Here's how the part is built. I have some questions about the finished solid (model axes, mm). Round coordinates to 2 decimals unless told otherwise and drop trailing zeros. Loops run counter-clockwise (first coordinate to the right, second up) from the corner with the lowest first, then second, coordinate; pieces in that order, holes last. Notation, with made-up numbers: (-22.75, 50) -> (-13.75, 50) arc R17 ccw to (-13.75, 54) -> close; hole circle Ø1 at (12, 3). An arc over 180 degrees is marked (long way). Use CSV: the item, a comma, the result in double quotes. Start each with the question number.
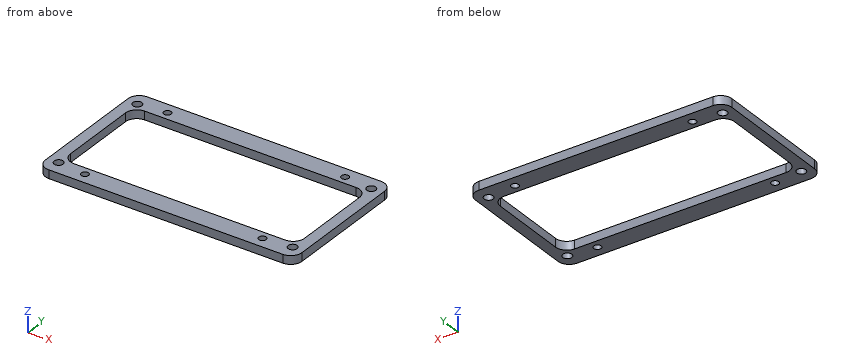
from build123d import *

# Parameters (mm, degrees)
SKETCH_1_W          = 91
SKETCH_1_H          = 50
SKETCH_1_W_2        = 83
SKETCH_1_H_2        = 36
EXTRUDE_1_DEPTH     = 3
SKETCH_2_R          = 1.3
CUT_EXTRUDE_1_DEPTH = 3
SKETCH_3_R          = 1.6
CUT_EXTRUDE_2_DEPTH = 3
FILLET_1_R          = 4
SKETCH_4_W          = 30
SKETCH_4_H          = 35
EXTRUDE_2_DEPTH     = 3
SKETCH_5_R          = 1.25
CUT_EXTRUDE_3_DEPTH = 10
FILLET_2_R          = 3
SKETCH_6_W          = 18
SKETCH_6_H          = 27
CUT_EXTRUDE_4_DEPTH = 10
FILLET_3_R          = 2
SKETCH_7_W          = 38
SKETCH_7_H          = 10
SKETCH_7_R          = 1.6
EXTRUDE_3_DEPTH     = 3
FILLET_4_R          = 2
FILLET_5_R          = 2
SKETCH_8_W          = 42
SKETCH_8_H          = 10
CUT_EXTRUDE_5_DEPTH = 10
SKETCH_9_W          = 30
SKETCH_9_H          = 41
CUT_EXTRUDE_6_DEPTH = 10


with BuildPart() as part:
    # 草图1 → 凸台-拉伸1 (new body)
    with BuildSketch(Plane.XY):
        Rectangle(SKETCH_1_W, SKETCH_1_H)
        Rectangle(SKETCH_1_W_2, SKETCH_1_H_2, mode=Mode.SUBTRACT)
    extrude(amount=EXTRUDE_1_DEPTH)

    # 草图2 → 切除-拉伸1 (cut)
    with BuildSketch(Plane.XY.offset(3)):
        with Locations((31.5, 21)):
            Circle(SKETCH_2_R)
        with Locations((31.5, -21)):
            Circle(SKETCH_2_R)
        with Locations((-31.5, -21)):
            Circle(SKETCH_2_R)
        with Locations((-31.5, 21)):
            Circle(SKETCH_2_R)
    extrude(amount=-CUT_EXTRUDE_1_DEPTH, mode=Mode.SUBTRACT)

    # 草图3 → 切除-拉伸2 (cut)
    with BuildSketch(Plane.XY.offset(3)):
        with Locations((41.5, 20)):
            Circle(SKETCH_3_R)
        with Locations((41.5, -20)):
            Circle(SKETCH_3_R)
        with Locations((-41.5, -20)):
            Circle(SKETCH_3_R)
        with Locations((-41.5, 20)):
            Circle(SKETCH_3_R)
    extrude(amount=-CUT_EXTRUDE_2_DEPTH, mode=Mode.SUBTRACT)

    # 圆角1
    fillet_1_edges = [part.edges().sort_by_distance(p)[0] for p in [
        (41.5, -18, 1.5),
        (41.5, 18, 1.5),
        (-41.5, 18, 1.5),
        (-41.5, -18, 1.5),
        (45.5, -25, 1.5),
        (-45.5, -25, 1.5),
        (-45.5, 25, 1.5),
        (45.5, 25, 1.5),
    ]]
    fillet(fillet_1_edges, radius=FILLET_1_R)

    # 草图4 → 凸台-拉伸2 (add)
    with BuildSketch(Plane(origin=(0, 0, 0), x_dir=(-1, 0, 0), z_dir=(0, 0, -1))):
        with Locations((-60.5, 0)):
            Rectangle(SKETCH_4_W, SKETCH_4_H)
    extrude(amount=-EXTRUDE_2_DEPTH)

    # 草图5 → 切除-拉伸3 (cut)
    with BuildSketch(Plane(origin=(0, 0, 0), x_dir=(-1, 0, 0), z_dir=(0, 0, -1))):
        with Locations((-70.5, -12)):
            Circle(SKETCH_5_R)
        with Locations((-70.5, 12)):
            Circle(SKETCH_5_R)
    extrude(amount=-CUT_EXTRUDE_3_DEPTH, mode=Mode.SUBTRACT)

    # 圆角2
    fillet_2_edges = [part.edges().sort_by_distance(p)[0] for p in [
        (45.5, 17.5, 1.5),
        (45.5, -17.5, 1.5),
        (75.5, -17.5, 1.5),
        (75.5, 17.5, 1.5),
    ]]
    fillet(fillet_2_edges, radius=FILLET_2_R)

    # 草图6 → 切除-拉伸4 (cut)
    with BuildSketch(Plane(origin=(0, 0, 0), x_dir=(-1, 0, 0), z_dir=(0, 0, -1))):
        with Locations((-57.5, 0)):
            Rectangle(SKETCH_6_W, SKETCH_6_H)
    extrude(amount=-CUT_EXTRUDE_4_DEPTH, mode=Mode.SUBTRACT)

    # 圆角3
    fillet_3_edges = [part.edges().sort_by_distance(p)[0] for p in [
        (66.5, -13.5, 1.5),
        (66.5, 13.5, 1.5),
        (48.5, 13.5, 1.5),
        (48.5, -13.5, 1.5),
    ]]
    fillet(fillet_3_edges, radius=FILLET_3_R)

    # 草图7 → 凸台-拉伸3 (add)
    with BuildSketch(Plane(origin=(0, 0, 0), x_dir=(-1, 0, 0), z_dir=(0, 0, -1))):
        with Locations((0, 30)):
            Rectangle(SKETCH_7_W, SKETCH_7_H)
        with Locations((-16, 32)):
            Circle(SKETCH_7_R, mode=Mode.SUBTRACT)
        with Locations((16, 32)):
            Circle(SKETCH_7_R, mode=Mode.SUBTRACT)
        with Locations((0, -30)):
            Rectangle(SKETCH_7_W, SKETCH_7_H)
        with Locations((16, -32)):
            Circle(SKETCH_7_R, mode=Mode.SUBTRACT)
        with Locations((-16, -32)):
            Circle(SKETCH_7_R, mode=Mode.SUBTRACT)
    extrude(amount=-EXTRUDE_3_DEPTH)

    # 圆角4
    fillet_4_edges = [part.edges().sort_by_distance(p)[0] for p in [
        (19, 35, 1.5),
        (-19, 35, 1.5),
        (-19, -35, 1.5),
        (19, -35, 1.5),
    ]]
    fillet(fillet_4_edges, radius=FILLET_4_R)

    # 圆角5
    fillet_5_edges = [part.edges().sort_by_distance(p)[0] for p in [
        (19, 25, 1.5),
        (-19, 25, 1.5),
        (-19, -25, 1.5),
        (19, -25, 1.5),
    ]]
    fillet(fillet_5_edges, radius=FILLET_5_R)

    # 草图8 → 切除-拉伸5 (cut)
    with BuildSketch(Plane.XY.offset(3)):
        with Locations((0, 30)):
            Rectangle(SKETCH_8_W, SKETCH_8_H)
        with Locations((0, -30)):
            Rectangle(SKETCH_8_W, SKETCH_8_H)
    extrude(amount=-CUT_EXTRUDE_5_DEPTH, mode=Mode.SUBTRACT)

    # 草图9 → 切除-拉伸6 (cut)
    with BuildSketch(Plane.XY.offset(3)):
        with Locations((60.5, 0)):
            Rectangle(SKETCH_9_W, SKETCH_9_H)
    extrude(amount=-CUT_EXTRUDE_6_DEPTH, mode=Mode.SUBTRACT)


solid = part.part
Q1. I want a section at D-D, the plane x = -29. List the corners of the cut face in (y, z) for me, then the cut area to 3 significant figures.
Q2. I want a section at C-C, the plane z = 2. Count the separate pieces of the cut face and the enclosed holes in it, then the cut area to 3 significant figures.
Q3. I want a section at B-B, the plane y = 2. List the corners of the cut face in (x, z) for me.
Q4. I want a section at A-A, the plane x = 31.5. List the corners of the cut face in (y, z) for me, then the cut area to 3 significant figures.
Q5. Will this pin go through, and if not, where does the flat tip stop? pin 1 Ø1.9 at (x, y) = (-41.5, -20) entering from -Z.
Q6. I need wall thicknesses on line 1 along Y through (x, z) = (-31.5, 1.55); line 2 along Y through (x, z) = (9, 2.5); line 3 along X through (y, z) = (-3, 0.6). Which ranges of each line are inside material? Lowest first, please.
Values found:
1,outline,"(-25, 0) -> (-18, 0) -> (-18, 3) -> (-25, 3) -> close; (18, 0) -> (25, 0) -> (25, 3) -> (18, 3) -> close"
1,area,"42.0 mm2"
2,separate pieces,"1"
2,enclosed holes,"9"
2,area,"1,510 mm2"
3,outline,"(-45.5, 0) -> (-41.5, 0) -> (-41.5, 3) -> (-45.5, 3) -> close; (41.5, 0) -> (45.5, 0) -> (45.5, 3) -> (41.5, 3) -> close"
4,outline,"(-25, 0) -> (-22.3, 0) -> (-22.3, 3) -> (-25, 3) -> close; (-19.7, 0) -> (-18, 0) -> (-18, 3) -> (-19.7, 3) -> close; (18, 0) -> (19.7, 0) -> (19.7, 3) -> (18, 3) -> close; (22.3, 0) -> (25, 0) -> (25, 3) -> (22.3, 3) -> close"
4,area,"26.4 mm2"
5,pin 1,"through"
6,line 1,"-25 to -22.3, -19.7 to -18, 18 to 19.7, 22.3 to 25"
6,line 2,"-25 to -18, 18 to 25"
6,line 3,"-45.5 to -41.5, 41.5 to 45.5"
